Work out the finished part from the listing and answer in its coordinate system (mm). A direction names the side the tool comes from. Coordinates: 2 decimals unless noted, no trailing zeros. Order: outer loops, then holes, each group sorted by start corner. A loop starts at its lowest first (then second) coordinate and runs counter-clockwise, first axis right, second up. Notation, with made-up numbers: M 3,59.25 L 41,59.25 A20 cw 41,82.25 Z; hole C 8,53.25 d7. An arc over 180 degrees is marked long. Use a Markdown table: item, result.
from build123d import *

# Parameters (mm, degrees)
F0_W     = 40
F0_H     = 40
F0_W_2   = 38
F0_H_2   = 38
F1_DEPTH = 1990
F3_DEPTH = 100
F5_DEPTH = 99


with BuildPart() as f1:
    # F0 (on Top) → F1 (new body)
    with BuildSketch(Plane.XY):
        Rectangle(F0_W, F0_H)
        Rectangle(F0_W_2, F0_H_2, mode=Mode.SUBTRACT)
    extrude(amount=F1_DEPTH)

    # F2 (on face) → F3 (cut)
    with BuildSketch(Plane.YZ.offset(20)):
        Polygon((-20, 1950), (20, 1990), (-20, 1990), align=None)
    extrude(amount=-F3_DEPTH, mode=Mode.SUBTRACT)

    # F4 (on face) → F5 (cut)
    with BuildSketch(Plane.YZ.offset(20)):
        Polygon((-20, 0), (20, 0), (-20, 40), align=None)
    extrude(amount=-F5_DEPTH, mode=Mode.SUBTRACT)


solid = f1.part
1. Section C-C on z = 133.5 is taken. Determine the outline of the cut face in (x, y).
Answers below:
| item | result |
|---|---|
| outline | M -20,-20 L 20,-20 L 20,20 L -20,20 Z; hole M -19,-19 L 19,-19 L 19,19 L -19,19 Z |
2. For a pull along X with two mould halves and no side action, classify faces 1 (the face through (19, 0, 981)), 2 (the face through (20, 0, 981)), 3 (the face through (-19.2, -1.6, 1968.4)) as +X half, -X half, draft (parallel to the pull), parting line (faces both ways), or undercut.
Answers below:
| item | result |
|---|---|
| face 1 | undercut |
| face 2 | +X half |
| face 3 | draft |
3. Section B-B on x = -12.5 is taken. Determine the outline of the cut face in (y, z).
Answers below:
| item | result |
|---|---|
| outline | M -20,40 L -19,39 L -19,1951 L -20,1950 Z; M 19,1 L 20,0 L 20,1990 L 19,1989 Z |
4. Find the intervals of material crossed by probe 1 along Y at (x, z) = (-8, 116), in increasing order.
Answers below:
| item | result |
|---|---|
| probe 1 | -20 to -19, 19 to 20 |
5. Section A-A on y = -1 is taken. Determine the outline of the cut face in (x, z).
Answers below:
| item | result |
|---|---|
| outline | M -20,21 L -19,21 L -19,1969 L -20,1969 Z; M 19,21 L 20,21 L 20,1969 L 19,1969 Z |
6. For faces 4 (the face through (-20, 0, 981)), 5 (the face through (0, 19, 981)), determine the directions among +Z, -Z, +X, -X, +Y, -Y from which every point of the face is accessible in a straight line to the end or side of a thin tool.
Answers below:
| item | result |
|---|---|
| face 4 | +Z, -Z, -X, +Y, -Y |
| face 5 | +Z, -Z |
